Can you work these out from the model? Positions are in its coordinate system, mm. A direction names the side the tool comes from. Coordinates: 2 decimals unless noted, no trailing zeros. Loops run counter-clockwise (first coordinate to the right, second up) from the corner with the lowest first, then second, coordinate; pieces in that order, holes last. Notation, with made-up numbers: (88.25, -20) -> (95.25, -20) arc R28 cw to (95.25, 14) -> close; hole circle Ø1 at (9, -18.75). An arc over 180 degrees is marked (long way). Put each result on its own line as item: value. Start each with the question number.
Item 1: Will these pins go through, and if not, where does the flat tip stop? P1, Ø15, axis at x = -7, y = 42, coming from the -Z side; P2, Ø9, axis at x = 0, z = 0, coming from the +Y side.
Item 2: If we section it at B-B on x = 0: Please give me the cut outline in (y, z), plus the area to 3 significant figures.
Item 3: If we section it at A-A on z = -99.5: Please give me the cut outline in (x, y).
Item 4: If we section it at C-C on y = 32: State how many separate pieces and enclosed holes the cut face has, plus the area to 4 significant figures.
Item 5: We'd pull the mould along Z, two halves only. Please class faces 3 (the cylindrical face through (1.08, 34.51, 4.88)), 4 (the flat face through (0, 35, -59.5)), 5 (the flat face through (-35, 35, -70)): pulls with the +Z half, pulls with the -Z half, needs draft (parallel to the pull), parting line crosses it, or undercut.
Item 6: For faces 1 (the flat face through (25, 35, -89)), 2 (the cylindrical face through (-29.93, 36.5, -104.27)), which set-ups out of +Z, -Z, +X, -X, +Y, -Y let a thin tool reach every point of the face, with its end or its side?
Item 7: Please list where these lines run through material, in increasing order: L1, parallel to Z at x = 0, y = 40; L2, parallel to Y at x = 31.75, z = -99.5; L3, parallel to X at y = 53, z = -122. Write a range as from..to.
Autodesk Inventor part; units mm, degrees
ref_plane "YZ Plane" through (0, 0, 0) normal (1, 0, 0) x (0, 1, 0)
ref_plane "XZ Plane" through (0, 0, 0) normal (0, 1, 0) x (-1, 0, 0)
ref_plane "XY Plane" through (0, 0, 0) normal (0, 0, 1) x (1, 0, 0)
sketch "Sketch1" plane through (0, 0, 0) normal (0, 1, 0) x (-1, 0, 0)
  arc A0 (35, 0) -> (-35, 0) centre (0, 0) ccw
  line L0 (35, 0) -> (-35, 0) construction
  line L1 (-35, 0) -> (-35, -139.5)
  line L2 (-35, -139.5) -> (35, -139.5)
  line L3 (35, -139.5) -> (35, 0)
  arc A1 (-35, 0) -> (35, 0) centre (0, 0) ccw construction
  line L4 (-25, -139.5) -> (25, -139.5)
  line L5 (25, -139.5) -> (25, -59.5)
  line L6 (25, -59.5) -> (-25, -59.5)
  line L7 (-25, -59.5) -> (-25, -139.5)
  circle A2 centre (0, 0) radius 5
  point P0 (25, -139.5)
  dimension "d0" = 70
  dimension "d1" = 139.5
  dimension "d2" = 10
  dimension "d3" = 10
  dimension "d4" = 80
  dimension "d11" = 10
extrude "Extrusion1" add sketch "Sketch1" along normal blind 70 contours L3 L2 L5 L6 L7 L1 A0
sketch "Sketch2" plane through (35, 0, 0) normal (1, 0, 0) x (0, 0, -1)
  line L0 (0, 0) -> (139.5, 0)
  line L1 (139.5, 0) -> (139.5, 70)
  line L2 (0, 70) -> (139.5, 70)
  line L3 (0, 0) -> (0, 70)
  arc A0 (118.8649, 70) -> (118.8649, 0) centre (99.5, 35) ccw
  line L4 (99.5, 35) -> (139.5, 35)
  arc A1 (139.5, 35) -> (118.8649, 70) centre (99.5, 35) ccw
  arc A2 (118.8649, 0) -> (139.5, 35) centre (99.5, 35) ccw
  circle A3 centre (99.5, 35) radius 5
  point P0 (0, 0)
  dimension "d7" = 80
  dimension "d8" = 10
extrude "Extrusion2" cut sketch "Sketch2" against normal through all contours A2 L1 L0 | A3 | A1 L2 L1
fillet "Fillet1" radius 2 16 edges at (0, 70, 35) (-35, 70, -59.4325) (35, 70, -59.4325) (0, 0, 35) (-35, 0, -59.4325) (35, 0, -59.4325) (-25, 35, -139.5) (35, 35, -139.5) (25, 35, -139.5) (-35, 35, -139.5) (-25, 70, -89.1825) (0, 70, -59.5) (0, 0, -59.5) (25, 0, -89.1825) (25, 70, -89.1825) (-25, 0, -89.1825)
properties part number "Wirst1"
Solutions:
1. P1: z = -59.5
1. P2: through
2. outline: (0, -57.5) arc R2 ccw to (2, -59.5) -> (68, -59.5) arc R2 ccw to (70, -57.5) -> (70, -5) -> (0, -5) -> close; (0, 5) -> (70, 5) -> (70, 33) arc R2 ccw to (68, 35) -> (2, 35) arc R2 ccw to (0, 33) -> close
2. area: 5,910 mm^2
3. outline: (-35, 2) arc R2 ccw to (-33, 0) -> (-27, 0) arc R2 ccw to (-25, 2) -> (-25, 30) -> (-35, 30) -> close; (-35, 40) -> (-25, 40) -> (-25, 68) arc R2 ccw to (-27, 70) -> (-33, 70) arc R2 ccw to (-35, 68) -> close; (25, 2) arc R2 ccw to (27, 0) -> (33, 0) arc R2 ccw to (35, 2) -> (35, 30) -> (25, 30) -> close; (25, 40) -> (35, 40) -> (35, 68) arc R2 ccw to (33, 70) -> (27, 70) arc R2 ccw to (25, 68) -> close
4. separate pieces: 3
4. enclosed holes: 1
4. area: 7,445 mm^2
5. face 3: undercut
5. face 4: pulls with the -Z half
5. face 5: needs draft
6. face 1: -Z, +Y, -Y
6. face 2: +X, -X
7. L1: -59.5..-5, 5..35
7. L2: 0..30, 40..70
7. L3: -35..-25, 25..35
